Here's how the part is built. I have some questions about the finished solid (model axes, mm). Coordinates: 2 decimals unless noted, no trailing zeros. Write each loop counter-clockwise with the first axis right and the second up, starting at its lowest first coordinate (ties: lowest second). Pieces come first, ordered by that corner, then holes. Notation, with made-up numbers: (7, -23.75) -> (46, -23.75) arc R15 cw to (46, 1.25) -> close; hole circle Ø2 at (57, 72). An arc over 180 degrees is marked (long way). Use a Markdown table: item, result. Add a question column.
Item 1: Imagine slicing it at A-A, the plane y = 6.5. Write out the boundary of the cut face in (x, z), and give its area (3 significant figures).
Item 2: Imagine slicing it at C-C, the plane x = 10. Write out the boundary of the cut face in (y, z).
Item 3: If we mould it in two halves opening along X, with no side actions, what happens to faces 1 (the flat face through (-29.21, 11, -4)), 2 (the flat face through (0, 30, 292.1)), 3 (the flat face through (31.75, 14, 4)), 4 (the cylindrical face through (-21.399, 21.568, -4.089))? For each: pulls with the +X half, pulls with the -X half, needs draft (parallel to the pull), parting line crosses it, or undercut.
Item 4: If I drill on line 1 along X through (y, z) = (25, -99); line 2 along X through (y, z) = (2, 129); line 3 along Y through (x, z) = (-25, 61), over which ranges is the centre line in solid material (lowest first)? Write a range as from..to.
Item 5: Imagine slicing it at B-B, the plane z = 244. Write out the boundary of the cut face in (x, y).
Item 6: Will this pin go through, and if not, where does the flat tip stop? pin 1 Ø13 at (x, z) = (0, 52) entering from -Y.
```python
from build123d import *

# Parameters (mm, degrees)
SKETCH1_W           = 63.5
SKETCH1_H           = 63.5
SKETCH1_R           = 3
BOSS_EXTRUDE1_DEPTH = 292.1
FILLET1_R           = 2.54
SHELL1_START        = -292.1
SHELL1_DEPTH        = 584.2
SKETCH3_W           = 63.665273771
SKETCH3_H           = 31.75
CUT_EXTRUDE2_DEPTH  = 586.923002621


# Read off the part's stored shape, not the designer's step: Shell1
with BuildPart() as part:
    # Sketch1 → Boss-Extrude1 (new, symmetric)
    with BuildSketch(Plane.XY):
        Rectangle(SKETCH1_W, SKETCH1_H)
        with Locations((-25.4, 25.4)):
            Circle(SKETCH1_R, mode=Mode.SUBTRACT)
        with Locations(Location((25.4, -25.4, 0), (0, 0, 180))):
            Circle(SKETCH1_R, mode=Mode.SUBTRACT)
        with Locations(Location((-25.4, -25.4, 0), (0, 0, 180))):
            Circle(SKETCH1_R, mode=Mode.SUBTRACT)
        with Locations(Location((25.4, 25.4, 0), (0, 0, 180))):
            Circle(SKETCH1_R, mode=Mode.SUBTRACT)
    extrude(amount=BOSS_EXTRUDE1_DEPTH, both=True)

    # Fillet1
    fillet1_edges = [part.edges().sort_by_distance(p)[0] for p in [
        (31.75, -31.75, 0),
        (-31.75, -31.75, 0),
        (-31.75, 31.75, 0),
        (31.75, 31.75, 0),
    ]]
    fillet(fillet1_edges, radius=FILLET1_R)

    # Shell1 outline → Shell1 (cut)
    with BuildSketch(Plane.XY.offset(SHELL1_START)):
        with BuildLine():
            Line((29.21, -21.378122329), (29.21, 21.378122329))
            ThreePointArc((29.21, 21.378122329), (21.482628432, 21.482628432), (21.378122329, 29.21))
            Line((21.378122329, 29.21), (-21.378122329, 29.21))
            ThreePointArc((-21.378122329, 29.21), (-21.482628432, 21.482628432), (-29.21, 21.378122329))
            Line((-29.21, 21.378122329), (-29.21, -21.378122329))
            ThreePointArc((-29.21, -21.378122329), (-21.482628432, -21.482628432), (-21.378122329, -29.21))
            Line((-21.378122329, -29.21), (21.378122329, -29.21))
            ThreePointArc((21.378122329, -29.21), (21.482628432, -21.482628432), (29.21, -21.378122329))
        make_face()
    extrude(amount=SHELL1_DEPTH, mode=Mode.SUBTRACT)

    # Sketch3 → Cut-Extrude2 (cut, through all)
    with BuildSketch(Plane.XY.offset(292.1)):
        with Locations((0.082636885, -16.003852467)):
            Rectangle(SKETCH3_W, SKETCH3_H)
    extrude(amount=-CUT_EXTRUDE2_DEPTH, mode=Mode.SUBTRACT)


solid = part.part
```
Ans:
| question | item | result |
|---|---|---|
| 1 | outline | (-31.75, -292.1) -> (-29.21, -292.1) -> (-29.21, 292.1) -> (-31.75, 292.1) -> close; (29.21, -292.1) -> (31.75, -292.1) -> (31.75, 292.1) -> (29.21, 292.1) -> close |
| 1 | area | 2,970 mm^2 |
| 2 | outline | (29.21, -292.1) -> (31.75, -292.1) -> (31.75, 292.1) -> (29.21, 292.1) -> close |
| 3 | face 1 | undercut |
| 3 | face 2 | needs draft |
| 3 | face 3 | pulls with the +X half |
| 3 | face 4 | undercut |
| 4 | line 1 | x = -31.75..-28.37, -22.43..-19.87, 19.87..22.43, 28.37..31.75 |
| 4 | line 2 | x = -31.75..-29.21, 29.21..31.75 |
| 4 | line 3 | y = 19.87..22.43, 28.37..31.75 |
| 5 | outline | (-31.75, -0.13) -> (-29.21, -0.13) -> (-29.21, 21.38) arc R5.54 ccw to (-21.38, 29.21) -> (21.38, 29.21) arc R5.54 ccw to (29.21, 21.38) -> (29.21, -0.13) -> (31.75, -0.13) -> (31.75, 29.21) arc R2.54 ccw to (29.21, 31.75) -> (-29.21, 31.75) arc R2.54 ccw to (-31.75, 29.21) -> close; hole circle Ø6 at (-25.4, 25.4); hole circle Ø6 at (25.4, 25.4) |
| 6 | pin 1 | stops at y = 29.21 |
